from build123d import *

# Parameters (mm, degrees)
SKETCH_W            = 180.2
SKETCH_H            = 8
PAD_DEPTH           = 2
SKETCH001_W         = 3
SKETCH001_H         = 8
PAD001_DEPTH        = 10
SKETCH002_R         = 1.1
HOLE_DEPTH          = 180.201
HOLE001_D           = 3.2
HOLE001_CSINK_D     = 5
HOLE001_CSINK_ANGLE = 90


with BuildPart() as part:
    # Sketch → Pad (new body)
    with BuildSketch(Plane.XY):
        Rectangle(SKETCH_W, SKETCH_H)
    extrude(amount=PAD_DEPTH)

    # Sketch001 (on Face6 of Pad) → Pad001 (join)
    with BuildSketch(Plane.XY.offset(2)):
        with Locations((-88.6, 0)):
            Rectangle(SKETCH001_W, SKETCH001_H)
        with Locations((88.6, 0)):
            Rectangle(SKETCH001_W, SKETCH001_H)
    extrude(amount=PAD001_DEPTH)

    # Sketch002 → Hole (cut, through all)
    with BuildSketch(Plane.YZ.offset(90.1)):
        with Locations((0, 8.2)):
            Circle(SKETCH002_R)
    extrude(amount=-HOLE_DEPTH, mode=Mode.SUBTRACT)

    # Hole001 (through all)
    with Locations(Plane.XY.offset(2)):
        with Locations((-73.085, 0), (0, 0), (73.085, 0)):
            CounterSinkHole(HOLE001_D / 2, HOLE001_CSINK_D / 2, counter_sink_angle=HOLE001_CSINK_ANGLE)


solid = part.part
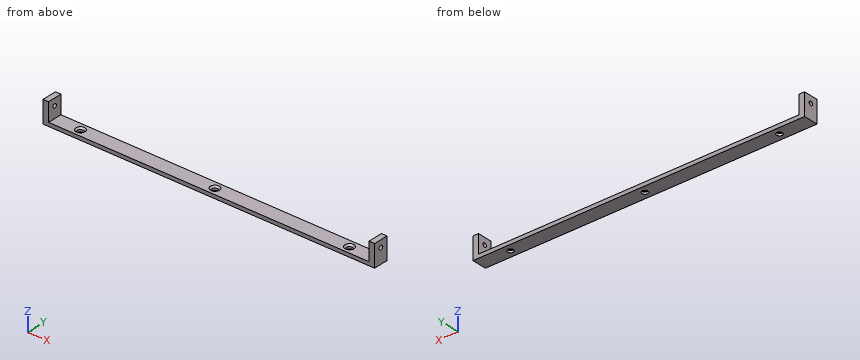
The model under review builds one solid part; all positions refer to its coordinate system, in mm. Coordinates: 2 decimals unless noted, no trailing zeros. Loops run counter-clockwise (first coordinate to the right, second up) from the corner with the lowest first, then second, coordinate; pieces in that order, holes last. Notation, with made-up numbers: M 36.5,39 L 49.5,39 A21 ccw 49.5,61 Z; hole C 36,-32 d5. An arc over 180 degrees is marked long. Put each result on its own line as item: value. Start each with the question number.
Q1. Add section C-C (x = 38). Write out the cut boundary in (y, z).
Q2. Add section A-A (z = 5.5). Write out the cut boundary in (x, y), and give its area (3 significant figures).
Q3. Clearance check with flat-ended pins moving along their axes: pin 1 (2.5 mm diameter, centred on y = 0.5, z = 7.5, fed in from +X); pin 2 (2.5 mm diameter, centred on x = -0.5, y = -2, fed in from +Z); pin 3 (4 mm diameter, centred on x = 73.085, y = 0, fed in from +Z). State where each tip first meets the part, or that it passes through.
Q4. Wall thickness on line 1 (X direction, y = 0, z = 0.8) (3 decimals); line 2 (X direction, y = -2, z = 3); line 3 (Z direction, x = -88.75, y = 0): over which ranges is each line inside the solid? List them lowest first.
Q5. Add section B-B (x = 0). Write out the cut boundary in (y, z), and give its area (3 significant figures).
Answers:
1. outline: M -4,0 L 4,0 L 4,2 L -4,2 Z
2. outline: M -90.1,-4 L -87.1,-4 L -87.1,4 L -90.1,4 Z; M 87.1,-4 L 90.1,-4 L 90.1,4 L 87.1,4 Z
2. area: 48.0 mm^2
3. pin 1: stops at x = 90.1
3. pin 2: stops at z = 2
3. pin 3: stops at z = 1.5
4. line 1: x = -90.1 to -74.685, -71.485 to -1.6, 1.6 to 71.485, 74.685 to 90.1
4. line 2: x = -90.1 to -87.1, 87.1 to 90.1
4. line 3: z = 0 to 7.1, 9.3 to 12
5. outline: M -4,0 L -1.6,0 L -1.6,1.1 L -2.5,2 L -4,2 Z; M 1.6,0 L 4,0 L 4,2 L 2.5,2 L 1.6,1.1 Z
5. area: 8.79 mm^2
